Autodesk Inventor part; units mm, degrees
ref_plane "YZ Plane" through (0, 0, 0) normal (1, 0, 0) x (0, 1, 0)
ref_plane "XZ Plane" through (0, 0, 0) normal (0, 1, 0) x (-1, 0, 0)
ref_plane "XY Plane" through (0, 0, 0) normal (0, 0, 1) x (1, 0, 0)
sketch "スケッチ1" plane through (0, 0, 0) normal (0, 0, 1) x (1, 0, 0)
  line L0 (-2.75, 1.5877) -> (0, 3.1754)
  line L1 (0, 3.1754) -> (2.75, 1.5877)
  line L2 (2.75, 1.5877) -> (2.75, -1.5877)
  line L3 (2.75, -1.5877) -> (0, -3.1754)
  line L4 (0, -3.1754) -> (-2.75, -1.5877)
  line L5 (-2.75, -1.5877) -> (-2.75, 1.5877)
  circle A0 centre (0, 0) radius 1.5
  dimension "d0" = 5.5
  dimension "d1" = 3
extrude "押し出し1" add sketch "スケッチ1" along normal blind 20 contours L0 L1 L2 L3 L4 L5 | A0
sketch "スケッチ2" plane through (0, 0, 20) normal (0, 0, 1) x (1, 0, 0)
  circle A0 centre (0, 0) radius 1.5
  dimension "d4" = 3
extrude "押し出し2" add sketch "スケッチ2" along normal blind 6
extrude "押し出し3" add sketch "スケッチ1" against normal blind 6 contours A0
properties part number "スペーサー　両雄ねじ　m3-20" material "アルミニウム 2014-T4"
CAD build for the part. Positions are in the model's coordinates, mm. A direction names the side the tool comes from. Round coordinates to 2 decimals unless told otherwise and drop trailing zeros. Write each loop counter-clockwise with the first axis right and the second up, starting at its lowest first coordinate (ties: lowest second). Pieces come first, ordered by that corner, then holes. Notation, with made-up numbers: (-13, 6) -> (2, 6) arc R24 cw to (2, 39) -> close; hole circle Ø7 at (-36.75, -37). An arc over 180 degrees is marked (long way). Answer as a JSON object with one key per item and string values.
(1) Which spindle directions (+Z, -Z, +X, -X, +Y, -Y) get a long thin tool onto all of the face, cutting with end or side? Do faces 1 (the face through (1.36, 2.39, 9.86)), 2 (the face through (-1.5, 0.07, -2.96)), 3 (the face through (-1.3, -1.4, 20)). Say none if no direction does.
Reported:
{"face 1": "+Z, -Z, +X, +Y", "face 2": "-Z", "face 3": "+Z"}
(2) Band-saw the part on B-B, the plane z = 12. List the corners of the cut face in (x, y).
Reported:
{"outline": "(-2.75, -1.59) -> (0, -3.18) -> (2.75, -1.59) -> (2.75, 1.59) -> (0, 3.18) -> (-2.75, 1.59) -> close"}
(3) Band-saw the part on A-A, the plane y = 0. List the corners of the cut face in (x, z).
Reported:
{"outline": "(-2.75, 0) -> (-1.5, 0) -> (-1.5, -6) -> (1.5, -6) -> (1.5, 0) -> (2.75, 0) -> (2.75, 20) -> (1.5, 20) -> (1.5, 26) -> (-1.5, 26) -> (-1.5, 20) -> (-2.75, 20) -> close"}
(4) Probe probe 1 along Z at (x, y) = (-1.4, 1); probe 2 along Y at (x, z) = (0.15, 9); probe 3 along X at (y, z) = (2.25, 14). List the from-to ranges inside material, lowest first. Write a range as [from, to].
Reported:
{"probe 1": "z = [0, 20]", "probe 2": "y = [-3.09, 3.09]", "probe 3": "x = [-1.6, 1.6]"}
(5) Band-saw the part on D-D, the plane y = 2.75. List the corners of the cut face in (x, z), then the cut area to 3 significant figures.
Reported:
{"outline": "(-0.74, 0) -> (0.74, 0) -> (0.74, 20) -> (-0.74, 20) -> close", "area": "29.5 mm^2"}
(6) Band-saw the part on C-C, the plane z = -2.5. List the corners of the cut face in (x, y).
Reported:
{"outline": "circle Ø3 at (0, 0)"}
